from build123d import *

# Parameters (mm, degrees)
SKETCH1_R           = 36
SKETCH1_R_2         = 27.5
BOSS_EXTRUDE1_DEPTH = 9
SKETCH2_R           = 33.5
SKETCH2_R_2         = 30
CUT_EXTRUDE1_DEPTH  = 1


with BuildPart() as part:
    # Sketch1 → Boss-Extrude1 (new body)
    with BuildSketch(Plane(origin=(0, 0, 0), x_dir=(1, 0, 0), z_dir=(0, 1, 0))):
        with Locations(Location((0, 0, 0), (0, 0, 270))):
            Circle(SKETCH1_R)
        with Locations(Location((0, 0, 0), (0, 0, 270))):
            Circle(SKETCH1_R_2, mode=Mode.SUBTRACT)
    extrude(amount=BOSS_EXTRUDE1_DEPTH)

    # Sketch2 → Cut-Extrude1 (cut)
    with BuildSketch(Plane(origin=(0, 9, 0), x_dir=(1, 0, 0), z_dir=(0, 1, 0))):
        with Locations(Location((0, 0, 0), (0, 0, 270))):
            Circle(SKETCH2_R)
        with Locations(Location((0, 0, 0), (0, 0, 270))):
            Circle(SKETCH2_R_2, mode=Mode.SUBTRACT)
    cut_extrude1 = extrude(amount=-CUT_EXTRUDE1_DEPTH, mode=Mode.SUBTRACT)

    # Mirror1: Cut-Extrude1 across plane
    add(cut_extrude1.mirror(Plane.ZX.offset(4.5)), mode=Mode.SUBTRACT)


solid = part.part
For this review, take the finished solid that the model builds, in its own axes (mm). A direction names the side the tool comes from. Give positions to 0.01 mm unless a question says otherwise; leave off trailing zeros. Loops run counter-clockwise (first coordinate to the right, second up) from the corner with the lowest first, then second, coordinate; pieces in that order, holes last. Notation, with made-up numbers: M 29.5,10 L 87.5,10 A26 cw 87.5,48 Z; hole C 11,-6.75 d2. An arc over 180 degrees is marked long. Put each result on its own line as item: value. Start each with the question number.
(1) Wall thickness on L1, parallel to X at y = 8.4, z = 0; L2, parallel to Z at x = 1, y = 4.5; L3, parallel to X at y = 6.75, z = 0: over which ranges is each line inside the solid? List them lowest first.
(2) The part is to be moulded in two halves that separate along Z. For faces 1 (the cylindrical face through (-24.397, 4.437, 12.69)), 2 (the flat face through (-24, 0, 24)), 3 (the cylindrical face through (10.81, 4.44, 34.34)), 4 (the cylindrical face through (1.32, 8.51, -29.97)), say which applies: +Z half, -Z half, draft (parallel to the pull), parting line (faces both ways), or undercut.
(3) Add section A-A, the plane z = 0. Write out the cut boundary in (x, y).
(4) Add section B-B, the plane x = 0. Write out the cut boundary in (y, z).
(5) Machinability: for faces 5 (the cylindrical face through (1.32, 0.49, -29.97)), 6 (the cylindrical face through (-29.7, 8.5, 15.5)), 7 (the flat face through (-24, 9, 24)), which of the approach directions +Z, -Z, +X, -X, +Y, -Y give a long, thin tool a straight path to every point of the face, cutting with its end or side? Answer none if there is none.
(6) Add section C-C, the plane y = 5. Write out the cut boundary in (x, z).
(7) For pin 1 (4 mm diameter, centred on x = 19, y = 3, fed in from +Z); pin 2 (5 mm diameter, centred on y = 1.5, z = 1, fed in from +X); pin 3 (1 mm diameter, centred on x = -6.5, y = 4, fed in from -Z), all flat-tipped, find the tip position at first contact; note any pin that passes through.
Result:
1. L1: x = -36 to -33.5, -30 to -27.5, 27.5 to 30, 33.5 to 36
1. L2: z = -35.99 to -27.48, 27.48 to 35.99
1. L3: x = -36 to -27.5, 27.5 to 36
2. face 1: undercut
2. face 2: draft
2. face 3: parting line
2. face 4: undercut
3. outline: M -36,0 L -33.5,0 L -33.5,1 L -30,1 L -30,0 L -27.5,0 L -27.5,9 L -30,9 L -30,8 L -33.5,8 L -33.5,9 L -36,9 Z; M 27.5,0 L 30,0 L 30,1 L 33.5,1 L 33.5,0 L 36,0 L 36,9 L 33.5,9 L 33.5,8 L 30,8 L 30,9 L 27.5,9 Z
4. outline: M 0,-36 L 9,-36 L 9,-33.5 L 8,-33.5 L 8,-30 L 9,-30 L 9,-27.5 L 0,-27.5 L 0,-30 L 1,-30 L 1,-33.5 L 0,-33.5 Z; M 0,27.5 L 9,27.5 L 9,30 L 8,30 L 8,33.5 L 9,33.5 L 9,36 L 0,36 L 0,33.5 L 1,33.5 L 1,30 L 0,30 Z
5. face 5: -Y
5. face 6: +Y
5. face 7: +Z, -Z, +X, -X, +Y
6. outline: C 0,0 d72; hole C 0,0 d55
7. pin 1: stops at z = 31.73
7. pin 2: stops at x = 36
7. pin 3: stops at z = -35.5
